from build123d import *

# Parameters (mm, degrees)
SKETCH1_R           = 42.5
BOSS_EXTRUDE1_DEPTH = 40
SKETCH2_R           = 2
BOSS_EXTRUDE2_DEPTH = 15
SKETCH3_R           = 2
BOSS_EXTRUDE3_DEPTH = 30


with BuildPart() as part:
    # Sketch1 → Boss-Extrude1 (new body, symmetric)
    with BuildSketch(Plane(origin=(0, 0, 0), x_dir=(0, 0, -1), z_dir=(1, 0, 0))):
        Circle(SKETCH1_R)
    extrude(amount=BOSS_EXTRUDE1_DEPTH, both=True)

    # Sketch2 → Boss-Extrude2 (add)
    with BuildSketch(Plane.ZY.offset(40)):
        with Locations((-15.290703643, 5.288943408)):
            Circle(SKETCH2_R)
    extrude(amount=BOSS_EXTRUDE2_DEPTH)

    # Sketch3 → Boss-Extrude3 (add)
    with BuildSketch(Plane(origin=(0, 15.527284441, -44.890460433), x_dir=(-1, 0, 0), z_dir=(0, 0.326890199, -0.945062325))):
        with Locations((-30, -35.619517122)):
            Circle(SKETCH3_R)
    extrude(amount=-BOSS_EXTRUDE3_DEPTH)


solid = part.part
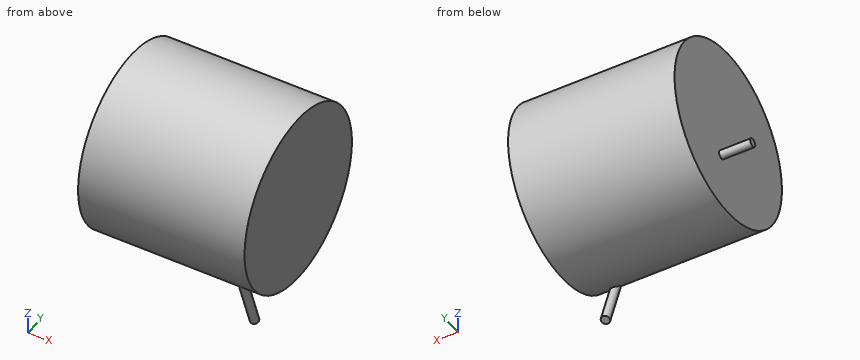
Geometry: final body of the model. Coordinates: model frame, mm. Give positions to 0.01 mm unless a question says otherwise; leave off trailing zeros. Write each loop counter-clockwise with the first axis right and the second up, starting at its lowest first coordinate (ties: lowest second). Pieces come first, ordered by that corner, then holes. Notation, with made-up numbers: M -26.75,28.25 L -17.75,28.25 A18 ccw -17.75,33.25 Z; hole C 26,-18.5 d6. An arc over 180 degrees is marked long. Answer in a Markdown table with one row per item. Add a question column.
(1) Ray query, line 1 (X direction, y = 19, z = 21.5); line 2 (Y direction, x = -33, z = -1); line 3 (Z direction, x = 15.5, y = 1.5). Return the intervals inside material, ascending.
(2) Section B-B on z = 0. Return loops of the section in (x, y).
(3) First-contact query: pin 1 (12 mm diameter, centred on x = 26.5, z = -32, fed in from -Y); pin 2 (8 mm diameter, centred on x = 24.5, y = -20, fed in from -Z); pin 3 (2 mm diameter, centred on x = -33, z = 0, fed in from +Y); pin 4 (5 mm diameter, centred on x = 16.5, y = 0.5, fed in from +Z). Flat tips, straight axial feed; report the tip coordinate or a pass-through.
(4) Section A-A on x = -27.5. Return loops of the section in (y, z).
Result set:
| question | item | result |
|---|---|---|
| 1 | line 1 | x = -40 to 40 |
| 1 | line 2 | y = -42.49 to 42.49 |
| 1 | line 3 | z = -42.47 to 42.47 |
| 2 | outline | M -40,-42.5 L 40,-42.5 L 40,42.5 L -40,42.5 Z |
| 3 | pin 1 | stops at y = -33.62 |
| 3 | pin 2 | stops at z = -56.94 |
| 3 | pin 3 | stops at y = 42.5 |
| 3 | pin 4 | stops at z = 42.5 |
| 4 | outline | C 0,0 d85 |
